```python
from build123d import *

# Parameters (mm, degrees)
BOSS_EXTRUDE1_DEPTH      = 3
SKETCH2_R                = 1.7
CUT_EXTRUDE1_DEPTH       = 3
BOSS_EXTRUDE2_DEPTH      = 3
BOSS_EXTRUDE2_DEPTH_BACK = 20
CUT_EXTRUDE2_DEPTH       = 17
SKETCH6_W                = 1.27
SKETCH6_H                = 5.08
BOSS_EXTRUDE3_DEPTH      = 10
FILLET1_R                = 0.508


with BuildPart() as part:
    # Sketch1 → Boss-Extrude1 (new body)
    with BuildSketch(Plane.XY):
        with BuildLine():
            Line((24, 22), (34.679465326, 15.221429328))
            ThreePointArc((34.679465326, 15.221429328), (37, 11), (34.679465326, 6.778570672))
            Line((34.679465326, 6.778570672), (24, 0))
            Line((24, 0), (0, 0))
            Line((0, 0), (-10.679465326, 6.778570672))
            ThreePointArc((-10.679465326, 6.778570672), (-13, 11), (-10.679465326, 15.221429328))
            Line((-10.679465326, 15.221429328), (0, 22))
            Line((0, 22), (24, 22))
        make_face()
    extrude(amount=BOSS_EXTRUDE1_DEPTH)

    # Sketch2 → Cut-Extrude1 (cut)
    with BuildSketch(Plane.XY.offset(3)):
        with Locations((32, 11)):
            Circle(SKETCH2_R)
        with Locations((-8, 11)):
            Circle(SKETCH2_R)
    extrude(amount=-CUT_EXTRUDE1_DEPTH, mode=Mode.SUBTRACT)

    # Sketch3 → Boss-Extrude2 (add, two sides: drawn at the far end of the back side and taken through both)
    with BuildSketch(Plane.XY.offset(3).offset(-BOSS_EXTRUDE2_DEPTH_BACK)):
        with BuildLine():
            Line((2, 22), (22, 22))
            ThreePointArc((22, 22), (25.535533906, 20.535533906), (27, 17))
            Line((27, 17), (27, 5))
            ThreePointArc((27, 5), (25.535533906, 1.464466094), (22, 0))
            Line((22, 0), (2, 0))
            ThreePointArc((2, 0), (-1.535533906, 1.464466094), (-3, 5))
            Line((-3, 5), (-3, 17))
            ThreePointArc((-3, 17), (-1.535533906, 20.535533906), (2, 22))
        make_face()
    extrude(amount=BOSS_EXTRUDE2_DEPTH + BOSS_EXTRUDE2_DEPTH_BACK)

    # Sketch5 → Cut-Extrude2 (cut)
    with BuildSketch(Plane.XY.offset(6)):
        Polygon((5, 19), (19, 19), (24, 14), (24, 3), (0, 3), (0, 14), align=None)
    extrude(amount=-CUT_EXTRUDE2_DEPTH, mode=Mode.SUBTRACT)

    # Sketch6 → Boss-Extrude3 (add)
    with BuildSketch(Plane.XY.offset(-11)):
        with Locations((12.058361068, 15.19)):
            Rectangle(SKETCH6_W, SKETCH6_H)
        with Locations((18.285, 7.57)):
            Rectangle(SKETCH6_W, SKETCH6_H)
        with Locations((5.715, 7.57)):
            Rectangle(SKETCH6_W, SKETCH6_H)
    extrude(amount=BOSS_EXTRUDE3_DEPTH)

    # Fillet1
    fillet1_edges = [part.edges().sort_by_distance(p)[0] for p in [
        (18.92, 7.57, -1),
        (18.285, 10.11, -1),
        (17.65, 7.57, -1),
        (18.285, 5.03, -1),
        (6.35, 7.57, -1),
        (5.715, 10.11, -1),
        (5.08, 7.57, -1),
        (5.715, 5.03, -1),
        (12.693361068, 15.19, -1),
        (12.058361068, 17.73, -1),
        (11.423361068, 15.19, -1),
        (12.058361068, 12.65, -1),
    ]]
    fillet(fillet1_edges, radius=FILLET1_R)


solid = part.part
```
Could you check a few things on this model? Use its own coordinates, in mm. A direction names the side the tool comes from. Round coordinates to 2 decimals unless told otherwise and drop trailing zeros. Loops run counter-clockwise (first coordinate to the right, second up) from the corner with the lowest first, then second, coordinate; pieces in that order, holes last. Notation, with made-up numbers: (-37.75, -11.5) -> (-6.75, -11.5) arc R13 cw to (-6.75, -4.5) -> close; hole circle Ø4 at (-17, 36.25). An arc over 180 degrees is marked (long way). One line per question, with ' | ' between items.
(1) If we section it at A-A on z = -2.75: List the corners of the cut face in (x, y) for me, and give its area (3 significant figures).
Model answer:
outline: (-3, 5) arc R5 ccw to (2, 0) -> (22, 0) arc R5 ccw to (27, 5) -> (27, 17) arc R5 ccw to (22, 22) -> (2, 22) arc R5 ccw to (-3, 17) -> close; (5.08, 5.03) -> (6.35, 5.03) -> (6.35, 10.11) -> (5.08, 10.11) -> close; (11.42, 12.65) -> (12.69, 12.65) -> (12.69, 17.73) -> (11.42, 17.73) -> close; (17.65, 5.03) -> (18.92, 5.03) -> (18.92, 10.11) -> (17.65, 10.11) -> close; hole (0, 3) -> (24, 3) -> (24, 14) -> (19, 19) -> (5, 19) -> (0, 14) -> close | area: 299 mm^2
(2) If we section it at B-B on y = 11: List the corners of the cut face in (x, z) for me, and give its area (3 significant figures).
Model answer:
outline: (-13, 0) -> (-9.7, 0) -> (-9.7, 3) -> (-13, 3) -> close; (-6.3, 0) -> (-3, 0) -> (-3, -17) -> (27, -17) -> (27, 0) -> (30.3, 0) -> (30.3, 3) -> (27, 3) -> (27, 6) -> (24, 6) -> (24, -11) -> (0, -11) -> (0, 6) -> (-3, 6) -> (-3, 3) -> (-6.3, 3) -> close; (33.7, 0) -> (37, 0) -> (37, 3) -> (33.7, 3) -> close | area: 322 mm^2
(3) For faces 1 (the face through (-2, 20, 4)), 2 (the face through (0, 8, -2)), 3 (the face through (-1, 1, 4)), 4 (the face through (26, 2, -9)), which set-ups out of +Z, -Z, +X, -X, +Y, -Y let a thin tool reach every point of the face, with its end or its side?
Model answer:
face 1: +Z, -X, +Y | face 2: +Z | face 3: +Z, -X, -Y | face 4: -Z, +X, -Y
(4) If we section it at C-C on x = 32: List the corners of the cut face in (y, z) for me.
Model answer:
outline: (5.08, 0) -> (9.3, 0) -> (9.3, 3) -> (5.08, 3) -> close; (12.7, 0) -> (16.92, 0) -> (16.92, 3) -> (12.7, 3) -> close
(5) If I drill on probe 1 along X at (y, z) = (12.75, -2.75); probe 2 along X at (y, z) = (10.75, 5); probe 3 along X at (y, z) = (5.75, -3.25), over which ranges is the centre line in solid material (lowest first)?
Model answer:
probe 1: x = -3 to 0, 11.42 to 12.69, 24 to 27 | probe 2: x = -3 to 0, 24 to 27 | probe 3: x = -3 to 0, 5.08 to 6.35, 17.65 to 18.92, 24 to 27
(6) If we section it at D-D on z = -14.25: List the corners of the cut face in (x, y) for me.
Model answer:
outline: (-3, 5) arc R5 ccw to (2, 0) -> (22, 0) arc R5 ccw to (27, 5) -> (27, 17) arc R5 ccw to (22, 22) -> (2, 22) arc R5 ccw to (-3, 17) -> close
(7) Thinking about a two-plate mould opening in Y: for faces 5 (the face through (25, 21, 4)), 6 (the face through (27, 11, 4)), 7 (the face through (24, 9, -2)), 8 (the face through (5.08, 8, -6)), which applies, released by +Y, released by -Y, zero draft, split by the parting line, or undercut?
Model answer:
face 5: released by +Y | face 6: zero draft | face 7: undercut | face 8: undercut
(8) For pin 1 Ø2 at (x, y) = (32, 11) entering from -Z; pin 2 Ø5 at (x, z) = (-3, -12.5) entering from +Y; pin 3 Ø10 at (y, z) = (19, -10) entering from +X; pin 4 Ø4 at (y, z) = (15.5, 1) entering from -X, each with a flat end and sliding along its axis, tell me the tip position at first contact or that it passes through.
Model answer:
pin 1: passes through | pin 2: stops at y = 21.33 | pin 3: stops at x = 27 | pin 4: stops at x = -12.33
